The listing builds one solid part. Answer for the finished solid, in the listing's coordinates (mm). Round coordinates to 2 decimals unless told otherwise and drop trailing zeros. Order: outer loops, then holes, each group sorted by start corner. A loop starts at its lowest first (then second) coordinate and runs counter-clockwise, first axis right, second up. Notation, with made-up numbers: (72, 18) - (95, 18) arc R26 cw to (95, 36) - close; hole circle Ø3 at (78, 62). An arc over 180 degrees is marked (long way). One line per item, written item: value. Start each with the question number.
1. Section B-B, the plane z = 5.5 is taken. Give the vertices of the cut face in (x, y), then the cut area to 3 significant figures.
2. Section A-A, the plane x = 0 is taken. Give the vertices of the cut face in (y, z), then the cut area to 3 significant figures.
3. Flat-ended cylindrical pins translate along their axes: P1, Ø1.7, axis at x = 0, y = 0, coming from the -Z side; P2, Ø1, axis at y = 2.5, z = 12, coming from the -X side; P3, Ø1, axis at y = -2.5, z = 13.5, coming from the +X side. Find the tip coordinate at first contact, or state that the pin passes through.
4. Straight lines are drawn through the part: line 1 (X direction, y = 0, z = 22); line 2 (Z direction, x = 0.5, y = 0). For each, find the intervals that lie inside material, in ascending order.
from build123d import *

# Parameters (mm, degrees)
F0_R      = 3.5
F1_DEPTH  = 25
F2_DEPTH  = 47
F3_R      = 1.65
F4_DEPTH  = 38
F5_R      = 1.13
F6_DEPTH  = 100
F6_TAPER  = -30
F8_R      = 1.03
F9_DEPTH  = 2
F9_TAPER  = 22.5
F10_R     = 0.75
F11_DEPTH = 5


# Not quite as in the source:
# - a feature names something its author has since deleted; it is built from what else it names


with BuildPart() as f1:
    # F0 (on Top) → F1 (new body)
    with BuildSketch(Plane.XY):
        Circle(F0_R)
    extrude(amount=F1_DEPTH)


with BuildPart() as f2:
    # F0 (on Top) → F2 (new body)
    with BuildSketch(Plane.XY):
        Circle(F0_R)
    extrude(amount=F2_DEPTH)


with BuildPart() as f4_tool:
    # F3 (on face) → F4 (new body)
    with BuildSketch(Plane(origin=(0, 0, 0), x_dir=(1, 0, 0), z_dir=(0, 0, -1))):
        Circle(F3_R)
    extrude(amount=-F4_DEPTH)


with BuildPart() as f1_1:
    add(f1.part)

    # F4: cut by f4_tool
    add(f4_tool.part, mode=Mode.SUBTRACT)


with BuildPart() as f2_1:
    add(f2.part)

    # F4: cut by f4_tool
    add(f4_tool.part, mode=Mode.SUBTRACT)


with BuildPart() as f6_tool:
    # F5 (on face) → F6 (new body)
    with BuildSketch(Plane.XY.offset(47)):
        Circle(F5_R)
    extrude(amount=-F6_DEPTH, taper=F6_TAPER)


with BuildPart() as f1_2:
    add(f1_1.part)

    # F6: intersect by f6_tool
    add(f6_tool.part, mode=Mode.INTERSECT)


with BuildPart() as f2_2:
    add(f2_1.part)

    # F6: intersect by f6_tool
    add(f6_tool.part, mode=Mode.INTERSECT)

    # F8 (on face) → F9 (cut)
    with BuildSketch(Plane.XY.offset(47)):
        Circle(F8_R)
    extrude(amount=-F9_DEPTH, taper=F9_TAPER, mode=Mode.SUBTRACT)

    # F10 (on face) → F11 (cut)
    with BuildSketch(Plane.XY.offset(47)):
        Circle(F10_R)
    extrude(amount=-F11_DEPTH, mode=Mode.SUBTRACT)


solid = f2_2.part
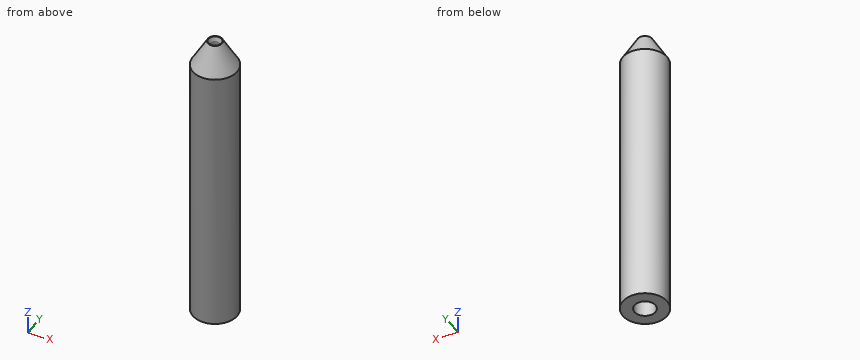
Answer list:
1. outline: circle Ø7 at (0, 0); hole circle Ø3.3 at (0, 0)
1. area: 29.9 mm²
2. outline: (-3.5, 0) - (-1.65, 0) - (-1.65, 38) - (1.65, 38) - (1.65, 0) - (3.5, 0) - (3.5, 42.9) - (1.13, 47) - (1.03, 47) - (0.75, 46.32) - (0.75, 42) - (-0.75, 42) - (-0.75, 46.32) - (-1.03, 47) - (-1.13, 47) - (-3.5, 42.9) - close
2. area: 186 mm²
3. P1: stops at z = 38
3. P2: stops at x = -2.87
3. P3: stops at x = 2.87
4. line 1: x = -3.5 to -1.65, 1.65 to 3.5
4. line 2: z = 38 to 42
